Source: three-view drawing plus pictorial views. Frame: mm from the lowest corner of the part. A direction names the side the tool comes from. Give positions to 0.01 mm unless a question says otherwise; leave off trailing zeros. Write each loop counter-clockwise with the first axis right and the second up, starting at its lowest first coordinate (ties: lowest second). Pieces come first, ordered by that corner, then holes.
Q1. Cut plane A-A on x = 104. Return the cut outline in (y, z), plus the area to 3 significant figures.
Q2. Cut plane D-D on x = 368.5. Return the cut outline in (y, z), plus the area to 3 significant figures.
Q3. Cut plane B-B on y = 32. Return the cut outline in (x, z), plus the area to 3 significant figures.
Q4. Cut plane C-C on z = 63. Return the cut outline in (x, y), plus the area to 3 significant figures.
Q5. Line query: L1, parallel to Y at x = 119, z = 444; L2, parallel to X at y = 92, z = 432; L3, parallel to X at y = 9, z = 216 (3 decimals). Output: solid intervals per line, ascending.
Q6. Draft query along Y for the marked faces 3, 4 and 5. Return one class per face: pulls with the +Y half, pulls with the -Y half, needs draft (parallel to the pull), parting line crosses it, or undercut.
Q7. Reachability of the marked faces 1 and 2 from +Z, -Z, +X, -X, +Y, -Y: full face, straight path, thin tool, end or side. Return the list, or none.
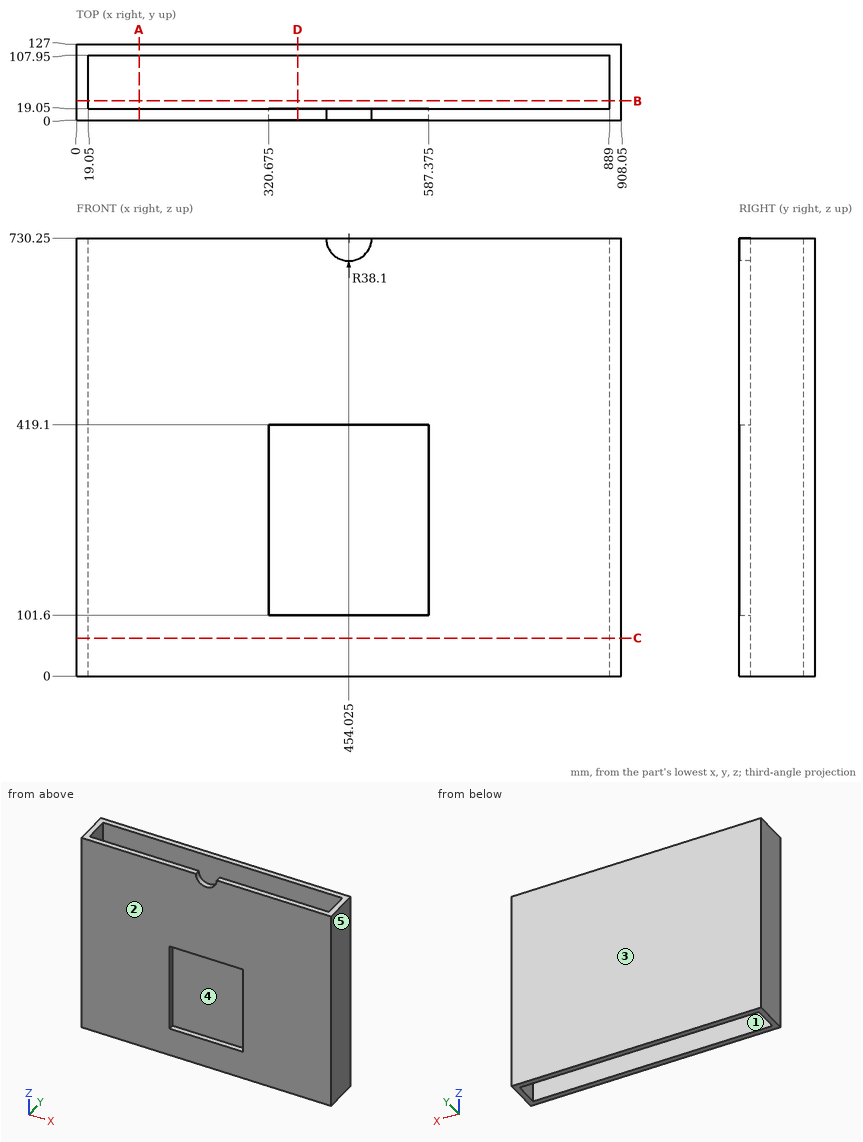
Data:
1. outline: (0, 0) - (19.05, 0) - (19.05, 730.25) - (0, 730.25) - close; (107.95, 0) - (127, 0) - (127, 730.25) - (107.95, 730.25) - close
1. area: 27,800 mm2
2. outline: (0, 0) - (19.05, 0) - (19.05, 101.6) - (0, 101.6) - close; (0, 419.1) - (19.05, 419.1) - (19.05, 730.25) - (0, 730.25) - close; (107.95, 0) - (127, 0) - (127, 730.25) - (107.95, 730.25) - close
2. area: 21,800 mm2
3. outline: (0, 0) - (19.05, 0) - (19.05, 730.25) - (0, 730.25) - close; (889, 0) - (908.05, 0) - (908.05, 730.25) - (889, 730.25) - close
3. area: 27,800 mm2
4. outline: (0, 0) - (908.05, 0) - (908.05, 127) - (0, 127) - close; hole (19.05, 19.05) - (889, 19.05) - (889, 107.95) - (19.05, 107.95) - close
4. area: 38,000 mm2
5. L1: y = 0 to 19.05, 107.95 to 127
5. L2: x = 0 to 19.05, 889 to 908.05
5. L3: x = 0 to 320.675, 587.375 to 908.05
6. face 3: pulls with the +Y half
6. face 4: undercut
6. face 5: needs draft
7. face 1: +Z, -Z
7. face 2: +Z, -Z, +X, -X, -Y
